Autodesk Inventor part; units mm, degrees
ref_plane "YZ Plane" through (0, 0, 0) normal (1, 0, 0) x (0, 1, 0)
ref_plane "XZ Plane" through (0, 0, 0) normal (0, 1, 0) x (-1, 0, 0)
ref_plane "XY Plane" through (0, 0, 0) normal (0, 0, 1) x (1, 0, 0)
sketch "Sketch1" plane through (0, 0, 0) normal (0, 1, 0) x (-1, 0, 0)
  circle A0 centre (0, 0) radius 11.43
  dimension "d0" = 22.86
extrude "Extrusion1" add sketch "Sketch1" along normal blind 6.35
sketch "Sketch2" plane through (0, 6.35, 0) normal (0, 1, 0) x (1, 0, 0)
  point P0 (0, 0)
  point P1 (0, 7.855)
  point P2 (0, -7.855)
  dimension "d3" = 15.7099
  dimension "d4" = 7.8549
  dimension "d21" = 7.8549
  dimension "d22" = 0
hole "Hole1" at (0, 6.35, -7.855) at (0, 6.35, 7.855) direction (0, -1, 0) diameter 3.4036 end through all counterbore diameter 5.715 counterbore depth 3.429
sketch "Sketch3" plane through (0, 6.35, 0) normal (0, 1, 0) x (1, 0, 0)
  circle A0 centre (0, 0) radius 3.175
  dimension "d12" = 6.35
extrude "Extrusion2" add sketch "Sketch3" along normal blind 19.05
sketch "Sketch4" plane through (0, 25.4, 0) normal (0, 1, 0) x (1, 0, 0)
  line L0 (1.5875, -1.5875) -> (-1.5875, -1.5875)
  line L1 (-1.5875, -1.5875) -> (-1.5875, 1.5875)
  line L2 (-1.5875, 1.5875) -> (1.5875, 1.5875)
  line L3 (1.5875, 1.5875) -> (1.5875, -1.5875)
  point P0 (0, 0)
  dimension "d15" = 3.175
  dimension "d16" = 3.175
  dimension "d17" = 1.5875
  dimension "d18" = 1.5875
extrude "Extrusion3" add sketch "Sketch4" along normal blind 10.16
properties part number "vex motor adaptor to tetrix"
CAD build for the part. Positions are in the model's coordinates, mm. A direction names the side the tool comes from. Round coordinates to 2 decimals unless told otherwise and drop trailing zeros. Write each loop counter-clockwise with the first axis right and the second up, starting at its lowest first coordinate (ties: lowest second). Pieces come first, ordered by that corner, then holes. Notation, with made-up numbers: M -39.5,43.5 L -29.5,43.5 A26 ccw -29.5,63.5 Z; hole C 87,65 d8. An arc over 180 degrees is marked long. Use a Markdown table: item, result. Add a question column.
1. Drill centre lines: probe 1 along Z at (x, y) = (0, 1.15); probe 2 along Y at (x, z) = (4.75, -1.5); probe 3 along Y at (x, z) = (1.75, 2). Where is each one in solid material? Low to high.
2. Flat gauge pins, fed straight in: P1, Ø5, axis at x = -1.5, y = 29.5, coming from the -Z side; P2, Ø8, axis at y = 28.5, z = -2.5, coming from the -X side (3 decimals); P3, Ø1.6, axis at y = 30.5, z = 0, coming from the +X side. Where does each tip first touch, or does it go through?
3. Slice it at A-A on x = 0. Give the number of separate pieces and of enclosed holes in the cut face, then the cut area to 3 significant figures.
4. Slice it at C-C on z = -7. Give the cut face in (x, y), then the cut area to 3 significant figures.
5. 3-axis set-ups, long thin cutter, end or side, ignore diameter. For faces 4 (the face through (0, 2.921, -6)), 5 (the face through (0, 30, 1.588)), 6 (the face through (0, 30, -1.588)): which of +Z, -Z, +X, -X, +Y, -Y reach the whole face in a straight line?
6. Pull direction X, two halves, no side cores. Call faces 1 (the face through (-1.588, 30, 0)), 2 (the face through (-0.075, 1.44, 6.155)), 3 (the face through (-10.902, 3.131, -3.433)): released by +X, released by -X, zero draft, split by the parting line, or undercut.
7. Slice it at D-D on y = 21. Give the cut face in (x, z) (3 decimals).
Reply:
| question | item | result |
|---|---|---|
| 1 | probe 1 | z = -11.43 to -9.56, -6.15 to 6.15, 9.56 to 11.43 |
| 1 | probe 2 | y = 0 to 6.35 |
| 1 | probe 3 | y = 0 to 25.4 |
| 2 | P1 | stops at z = -1.59 |
| 2 | P2 | stops at x = -3.175 |
| 2 | P3 | stops at x = 1.59 |
| 3 | separate pieces | 3 |
| 3 | enclosed holes | 0 |
| 3 | area | 239 mm^2 |
| 4 | outline | M -9.04,0 L -1.47,0 L -1.47,2.92 L -2.73,2.92 L -2.73,6.35 L -9.04,6.35 Z; M 1.47,0 L 9.04,0 L 9.04,6.35 L 2.73,6.35 L 2.73,2.92 L 1.47,2.92 Z |
| 4 | area | 87.5 mm^2 |
| 5 | face 4 | +Y |
| 5 | face 5 | +Z, +X, -X, +Y |
| 5 | face 6 | -Z, +X, -X, +Y |
| 6 | face 1 | released by -X |
| 6 | face 2 | undercut |
| 6 | face 3 | split by the parting line |
| 7 | outline | C 0,0 d6.35 |
